Source: CAD feature listing. Evaluate the final solid. Frame: model axes, mm. Round coordinates to 2 decimals unless told otherwise and drop trailing zeros. Order: outer loops, then holes, each group sorted by start corner. A loop starts at its lowest first (then second) coordinate and runs counter-clockwise, first axis right, second up. Notation, with made-up numbers: M 53.5,22 L 60.5,22 A23 ccw 60.5,42 Z; hole C -10,63.25 d3. An arc over 180 degrees is marked long. Use one line per item in the form item = value. Start each with the question number.
Q1. Pull-direction query (Z, two-part tool) for faces 1 (the cylindrical face through (35.683, -13.595, -3.248)), 2 (the cylindrical face through (36.048, -13.595, 32.316)), 3 (the cylindrical face through (-63.218, -13.595, -20.219)), 4 (the cylindrical face through (-63.22, -25.9, 5.69)); classes: pulls with the +Z half, pulls with the -Z half, needs draft (parallel to the pull), parting line crosses it, or undercut.
Q2. Section A-A (y = -9.5). Return the cut outline in (x, z), plus the area to 3 significant figures.
Q3. Section B-B (y = -1.75). Return the cut outline in (x, z).
Q4. Material intervals for probe 1 along Z at (x, y) = (12.5, -12.5); probe 2 along X at (y, z) = (-10, 6); probe 3 along X at (y, z) = (-5.25, 10), sorted ascending.
Q5. Contact query for a flat-ended pin moving along its axis: pin 1 (10 mm diameter, centred on y = -24, z = -14.5, fed in from +X). Output: stop coordinate, or through.
from build123d import *

# Parameters (mm, degrees)
F0_W         = 102.2414937615
F0_H         = 55.510988459
F0_R         = 18.1160237287
F1_DEPTH     = 27.432
F2_T1_DEPTH  = 92.0814937615
F2_T3_DEPTH  = 45.350988459
F2_T5_DEPTH  = 17.272
F2_S9_W      = 5.08
F2_S9_H      = 5.08
F2_T10_DEPTH = 5.08
F2_S15_W     = 5.08
F2_S15_H     = 5.08
F2_T16_DEPTH = 5.08
F2_S21_W     = 5.08
F2_S21_H     = 5.08
F2_T22_DEPTH = 5.08
F2_S27_W     = 5.08
F2_S27_H     = 5.08
F2_T28_DEPTH = 5.08
F2_S33_W     = 5.08
F2_S33_H     = 5.08
F2_T34_DEPTH = 5.08
F2_S39_W     = 5.08
F2_S39_H     = 5.08
F2_T40_DEPTH = 5.08
F2_S45_W     = 5.08
F2_S45_H     = 5.08
F2_T46_DEPTH = 5.08
F2_S51_W     = 5.08
F2_S51_H     = 5.08
F2_T52_DEPTH = 5.08


# Not quite as in the source:
# - a fillet or chamfer that OpenCascade refuses, or shapes differently, is made with other operations: its cross-section is extruded or revolved along the edge and cut away or added


with BuildPart() as f1:
    # F0 (on Front) → F1 (new body)
    with BuildSketch(Plane.XZ):
        with Locations((-13.5455615819, 6.0090096667)):
            Rectangle(F0_W, F0_H)
        with Locations((18.9486481249, 3.6901270505)):
            Circle(F0_R, mode=Mode.SUBTRACT)
    extrude(amount=F1_DEPTH)

    # F2: fillet of radius 5.08 on 15 edges, made by hand

    # F2_s2 → F2_t1 (cut)
    with BuildSketch(Plane.YZ.offset(-59.5863084626)):
        with BuildLine():
            ThreePointArc((-22.352, 33.7645038962), (-25.9441024484, 32.2766063447), (-27.432, 28.6845038962))
            Line((-27.432, 28.6845038962), (-27.432, 33.7645038962))
            Line((-27.432, 33.7645038962), (-22.352, 33.7645038962))
        make_face()
        with BuildLine():
            ThreePointArc((-22.352, -21.7464845628), (-25.9441024484, -20.2585870112), (-27.432, -16.6664845628))
            Line((-27.432, -16.6664845628), (-27.432, -21.7464845628))
            Line((-27.432, -21.7464845628), (-22.352, -21.7464845628))
        make_face()
        with BuildLine():
            ThreePointArc((-5.08, -21.7464845628), (-1.4878975516, -20.2585870112), (0, -16.6664845628))
            Line((0, -16.6664845628), (0, -21.7464845628))
            Line((0, -21.7464845628), (-5.08, -21.7464845628))
        make_face()
        with BuildLine():
            ThreePointArc((-5.08, 33.7645038962), (-1.4878975516, 32.2766063447), (0, 28.6845038962))
            Line((0, 28.6845038962), (0, 33.7645038962))
            Line((0, 33.7645038962), (-5.08, 33.7645038962))
        make_face()
    extrude(amount=F2_T1_DEPTH, mode=Mode.SUBTRACT)

    # F2_s4 → F2_t3 (cut)
    with BuildSketch(Plane.XY.offset(-16.6664845628)):
        with BuildLine():
            ThreePointArc((-64.6663084626, -22.352), (-63.178410911, -25.9441024484), (-59.5863084626, -27.432))
            Line((-59.5863084626, -27.432), (-64.6663084626, -27.432))
            Line((-64.6663084626, -27.432), (-64.6663084626, -22.352))
        make_face()
        with BuildLine():
            ThreePointArc((37.5751852989, -22.352), (36.0872877473, -25.9441024484), (32.4951852989, -27.432))
            Line((32.4951852989, -27.432), (37.5751852989, -27.432))
            Line((37.5751852989, -27.432), (37.5751852989, -22.352))
        make_face()
        with BuildLine():
            ThreePointArc((-64.6663084626, -5.08), (-63.178410911, -1.4878975516), (-59.5863084626, 0))
            Line((-59.5863084626, 0), (-64.6663084626, 0))
            Line((-64.6663084626, 0), (-64.6663084626, -5.08))
        make_face()
        with BuildLine():
            ThreePointArc((37.5751852989, -5.08), (36.0872877473, -1.4878975516), (32.4951852989, 0))
            Line((32.4951852989, 0), (37.5751852989, 0))
            Line((37.5751852989, 0), (37.5751852989, -5.08))
        make_face()
    extrude(amount=F2_T3_DEPTH, mode=Mode.SUBTRACT)

    # F2_s6 → F2_t5 (cut)
    with BuildSketch(Plane.XZ.offset(5.08)):
        with BuildLine():
            ThreePointArc((-64.6663084626, -16.6664845628), (-63.178410911, -20.2585870112), (-59.5863084626, -21.7464845628))
            Line((-59.5863084626, -21.7464845628), (-64.6663084626, -21.7464845628))
            Line((-64.6663084626, -21.7464845628), (-64.6663084626, -16.6664845628))
        make_face()
        with BuildLine():
            ThreePointArc((32.4951852989, -21.7464845628), (36.0872877473, -20.2585870112), (37.5751852989, -16.6664845628))
            Line((37.5751852989, -16.6664845628), (37.5751852989, -21.7464845628))
            Line((37.5751852989, -21.7464845628), (32.4951852989, -21.7464845628))
        make_face()
        with BuildLine():
            ThreePointArc((-59.5863084626, 33.7645038962), (-63.178410911, 32.2766063447), (-64.6663084626, 28.6845038962))
            Line((-64.6663084626, 28.6845038962), (-64.6663084626, 33.7645038962))
            Line((-64.6663084626, 33.7645038962), (-59.5863084626, 33.7645038962))
        make_face()
        with BuildLine():
            ThreePointArc((32.4951852989, 33.7645038962), (36.0872877473, 32.2766063447), (37.5751852989, 28.6845038962))
            Line((37.5751852989, 28.6845038962), (37.5751852989, 33.7645038962))
            Line((37.5751852989, 33.7645038962), (32.4951852989, 33.7645038962))
        make_face()
    extrude(amount=F2_T5_DEPTH, mode=Mode.SUBTRACT)


with BuildPart() as f2_tool8:
    # F2_s9 → F2_t10 (new body)
    with BuildSketch(Plane.XY.offset(28.6845038962)):
        with Locations((35.0351852989, -24.892)):
            Rectangle(F2_S9_W, F2_S9_H)
    extrude(amount=F2_T10_DEPTH)

    # F2_s11 → F2_t12 (revolve, cut)
    with BuildSketch(Plane(origin=(32.4951852989, -22.352, 28.6845038962), x_dir=(-0.7071067812, 0.7071067812, 0), z_dir=(0.7071067812, 0.7071067812, 0))):
        with BuildLine():
            ThreePointArc((0, -5.08), (5.08, 0), (0, 5.08))
            Line((0, 5.08), (0, -5.08))
        make_face()
    revolve(axis=Axis((32.4951852989, -22.352, 28.6845038962), (0, 0, 1)), mode=Mode.SUBTRACT)


with BuildPart() as f1_1:
    add(f1.part)

    # F2_t7: cut F2_tool8
    add(f2_tool8.part, mode=Mode.SUBTRACT)


with BuildPart() as f2_tool14:
    # F2_s15 → F2_t16 (new body)
    with BuildSketch(Plane.XY.offset(28.6845038962)):
        with Locations((-62.1263084626, -24.892)):
            Rectangle(F2_S15_W, F2_S15_H)
    extrude(amount=F2_T16_DEPTH)

    # F2_s17 → F2_t18 (revolve, cut)
    with BuildSketch(Plane(origin=(-59.5863084626, -22.352, 28.6845038962), x_dir=(0.7071067812, 0.7071067812, 0), z_dir=(0.7071067812, -0.7071067812, 0))):
        with BuildLine():
            ThreePointArc((0, -5.08), (5.08, 0), (0, 5.08))
            Line((0, 5.08), (0, -5.08))
        make_face()
    revolve(axis=Axis((-59.5863084626, -22.352, 28.6845038962), (0, 0, 1)), mode=Mode.SUBTRACT)


with BuildPart() as f1_2:
    add(f1_1.part)

    # F2_t13: cut F2_tool14
    add(f2_tool14.part, mode=Mode.SUBTRACT)


with BuildPart() as f2_tool20:
    # F2_s21 → F2_t22 (new body)
    with BuildSketch(Plane.YZ.offset(-59.5863084626)):
        with Locations((-24.892, -19.2064845628)):
            Rectangle(F2_S21_W, F2_S21_H)
    extrude(amount=-F2_T22_DEPTH)

    # F2_s23 → F2_t24 (revolve, cut)
    with BuildSketch(Plane(origin=(-59.5863084626, -22.352, -16.6664845628), x_dir=(0, 0.7071067812, 0.7071067812), z_dir=(0, -0.7071067812, 0.7071067812))):
        with BuildLine():
            ThreePointArc((0, -5.08), (5.08, 0), (0, 5.08))
            Line((0, 5.08), (0, -5.08))
        make_face()
    revolve(axis=Axis((-59.5863084626, -22.352, -16.6664845628), (-1, 0, 0)), mode=Mode.SUBTRACT)


with BuildPart() as f1_3:
    add(f1_2.part)

    # F2_t19: cut F2_tool20
    add(f2_tool20.part, mode=Mode.SUBTRACT)


with BuildPart() as f2_tool26:
    # F2_s27 → F2_t28 (new body)
    with BuildSketch(Plane.XY.offset(-16.6664845628)):
        with Locations((35.0351852989, -24.892)):
            Rectangle(F2_S27_W, F2_S27_H)
    extrude(amount=-F2_T28_DEPTH)

    # F2_s29 → F2_t30 (revolve, cut)
    with BuildSketch(Plane(origin=(32.4951852989, -22.352, -16.6664845628), x_dir=(-0.7071067812, 0.7071067812, 0), z_dir=(-0.7071067812, -0.7071067812, 0))):
        with BuildLine():
            ThreePointArc((0, -5.08), (5.08, 0), (0, 5.08))
            Line((0, 5.08), (0, -5.08))
        make_face()
    revolve(axis=Axis((32.4951852989, -22.352, -16.6664845628), (0, 0, -1)), mode=Mode.SUBTRACT)


with BuildPart() as f1_4:
    add(f1_3.part)

    # F2_t25: cut F2_tool26
    add(f2_tool26.part, mode=Mode.SUBTRACT)


with BuildPart() as f2_tool32:
    # F2_s33 → F2_t34 (new body)
    with BuildSketch(Plane.YZ.offset(-59.5863084626)):
        with Locations((-2.54, -19.2064845628)):
            Rectangle(F2_S33_W, F2_S33_H)
    extrude(amount=-F2_T34_DEPTH)

    # F2_s35 → F2_t36 (revolve, cut)
    with BuildSketch(Plane(origin=(-59.5863084626, -5.08, -16.6664845628), x_dir=(0, -0.7071067812, 0.7071067812), z_dir=(0, -0.7071067812, -0.7071067812))):
        with BuildLine():
            ThreePointArc((0, -5.08), (5.08, 0), (0, 5.08))
            Line((0, 5.08), (0, -5.08))
        make_face()
    revolve(axis=Axis((-59.5863084626, -5.08, -16.6664845628), (-1, 0, 0)), mode=Mode.SUBTRACT)


with BuildPart() as f1_5:
    add(f1_4.part)

    # F2_t31: cut F2_tool32
    add(f2_tool32.part, mode=Mode.SUBTRACT)


with BuildPart() as f2_tool38:
    # F2_s39 → F2_t40 (new body)
    with BuildSketch(Plane.XY.offset(-16.6664845628)):
        with Locations((35.0351852989, -2.54)):
            Rectangle(F2_S39_W, F2_S39_H)
    extrude(amount=-F2_T40_DEPTH)

    # F2_s41 → F2_t42 (revolve, cut)
    with BuildSketch(Plane(origin=(32.4951852989, -5.08, -16.6664845628), x_dir=(-0.7071067812, -0.7071067812, 0), z_dir=(0.7071067812, -0.7071067812, 0))):
        with BuildLine():
            ThreePointArc((0, -5.08), (5.08, 0), (0, 5.08))
            Line((0, 5.08), (0, -5.08))
        make_face()
    revolve(axis=Axis((32.4951852989, -5.08, -16.6664845628), (0, 0, -1)), mode=Mode.SUBTRACT)


with BuildPart() as f1_6:
    add(f1_5.part)

    # F2_t37: cut F2_tool38
    add(f2_tool38.part, mode=Mode.SUBTRACT)


with BuildPart() as f2_tool44:
    # F2_s45 → F2_t46 (new body)
    with BuildSketch(Plane.XY.offset(28.6845038962)):
        with Locations((35.0351852989, -2.54)):
            Rectangle(F2_S45_W, F2_S45_H)
    extrude(amount=F2_T46_DEPTH)

    # F2_s47 → F2_t48 (revolve, cut)
    with BuildSketch(Plane(origin=(32.4951852989, -5.08, 28.6845038962), x_dir=(-0.7071067812, -0.7071067812, 0), z_dir=(-0.7071067812, 0.7071067812, 0))):
        with BuildLine():
            ThreePointArc((0, -5.08), (5.08, 0), (0, 5.08))
            Line((0, 5.08), (0, -5.08))
        make_face()
    revolve(axis=Axis((32.4951852989, -5.08, 28.6845038962), (0, 0, 1)), mode=Mode.SUBTRACT)


with BuildPart() as f1_7:
    add(f1_6.part)

    # F2_t43: cut F2_tool44
    add(f2_tool44.part, mode=Mode.SUBTRACT)


with BuildPart() as f2_tool50:
    # F2_s51 → F2_t52 (new body)
    with BuildSketch(Plane.XY.offset(28.6845038962)):
        with Locations((-62.1263084626, -2.54)):
            Rectangle(F2_S51_W, F2_S51_H)
    extrude(amount=F2_T52_DEPTH)

    # F2_s53 → F2_t54 (revolve, cut)
    with BuildSketch(Plane(origin=(-59.5863084626, -5.08, 28.6845038962), x_dir=(0.7071067812, -0.7071067812, 0), z_dir=(-0.7071067812, -0.7071067812, 0))):
        with BuildLine():
            ThreePointArc((0, -5.08), (5.08, 0), (0, 5.08))
            Line((0, 5.08), (0, -5.08))
        make_face()
    revolve(axis=Axis((-59.5863084626, -5.08, 28.6845038962), (0, 0, 1)), mode=Mode.SUBTRACT)


with BuildPart() as f1_8:
    add(f1_7.part)

    # F2_t49: cut F2_tool50
    add(f2_tool50.part, mode=Mode.SUBTRACT)

    # F2_s55 → F2_t56 (revolve, cut)
    with BuildSketch(Plane.XY.offset(3.6901270505)):
        with BuildLine():
            ThreePointArc((37.0646718537, -22.352), (38.5525694052, -25.9441024484), (42.1446718537, -27.432))
            Line((42.1446718537, -27.432), (37.0646718537, -27.432))
            Line((37.0646718537, -27.432), (37.0646718537, -22.352))
        make_face()
    revolve(axis=Axis((18.9486481249, -27.432, 3.6901270505), (0, -1, 0)), mode=Mode.SUBTRACT)

    # F2_s57 → F2_t58 (revolve, cut)
    with BuildSketch(Plane.XY.offset(3.6901270505)):
        with BuildLine():
            ThreePointArc((37.0646718537, -5.08), (38.5525694052, -1.4878975516), (42.1446718537, 0))
            Line((42.1446718537, 0), (37.0646718537, 0))
            Line((37.0646718537, 0), (37.0646718537, -5.08))
        make_face()
    revolve(axis=Axis((18.9486481249, 0, 3.6901270505), (0, -1, 0)), mode=Mode.SUBTRACT)


solid = f1_8.part
Results list:
q1.face_1 = undercut
q1.face_2 = pulls with the +Z half
q1.face_3 = pulls with the -Z half
q1.face_4 = needs draft
q2.outline = M -64.67,-16.67 A5.08 ccw -59.59,-21.75 L 32.5,-21.75 A5.08 ccw 37.58,-16.67 L 37.58,28.68 A5.08 ccw 32.5,33.76 L -59.59,33.76 A5.08 ccw -64.67,28.68 Z; hole C 18.95,3.69 d36.23
q2.area = 4,620 mm2
q3.outline = M -63.42,-16.67 A3.84 ccw -59.59,-20.5 L 32.5,-20.5 A3.84 ccw 36.33,-16.67 L 36.33,-4.83 A19.36 cw long 36.33,12.21 L 36.33,28.68 A3.84 ccw 32.5,32.52 L -59.59,32.52 A3.84 ccw -63.42,28.68 Z
q4.probe_1 = -21.75 to -13.24, 20.62 to 33.76
q4.probe_2 = -64.67 to 0.98, 36.92 to 37.58
q4.probe_3 = -64.67 to 1.97, 35.93 to 37.58
q5.pin_1 = 37.58
